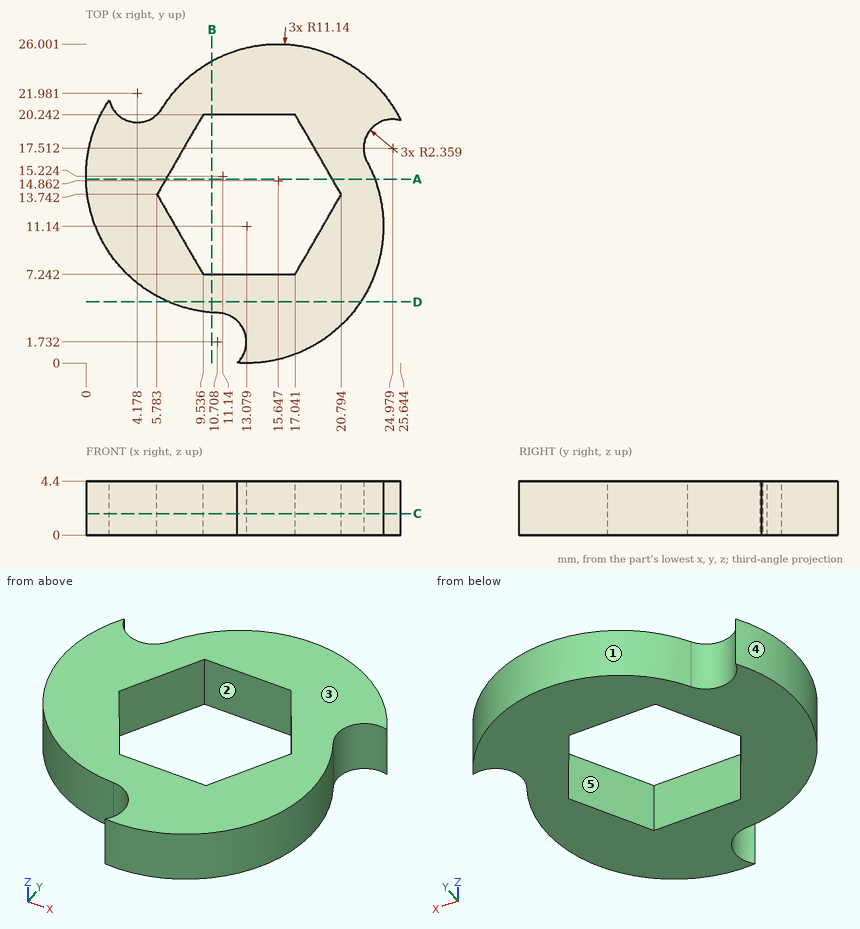
Drawing for the job (mm, zero at the part's lowest x, y, z). A direction names the side the tool comes from. Coordinates: 2 decimals unless noted, no trailing zeros. Order: outer loops, then holes, each group sorted by start corner. A loop starts at its lowest first (then second) coordinate and runs counter-clockwise, first axis right, second up. Notation, with made-up numbers: (51.5, 33.25) -> (55.5, 33.25) arc R11 ccw to (55.5, 50.25) -> close; hole circle Ø4 at (46, 22). An arc over 180 degrees is marked (long way). One line per item, written item: value.
(1) Slice it at B-B, the plane x = 10.25. List the corners of the cut face in (y, z).
Checked values:
outline: (4.12, 0) -> (7.24, 0) -> (7.24, 4.4) -> (4.12, 4.4) -> close; (20.24, 0) -> (24.61, 0) -> (24.61, 4.4) -> (20.24, 4.4) -> close
(2) Tool access for the marked faces 1 and 2: list every direction of +Z, -Z, +X, -X, +Y, -Y with a clear straight run to the whole face (end or side of a thin tool).
Checked values:
face 1: +Z, -Z, +Y
face 2: +Z, -Z
(3) Probe line 1 (Y direction, x = 16, z = 1) (1 decimal); line 2 (X direction, y = 12.5, z = 2.85) (1 decimal); line 3 (Y direction, x = 6, z = 0.9) (1 decimal). List the from-to ranges inside material, lowest first. Write a range as [from, to].
Checked values:
line 1: [0.4, 7.2], [20.2, 26]
line 2: [0.3, 6.5], [20.1, 24.1]
line 3: [5.3, 13.4], [14.1, 20.5]
(4) Slice it at D-D, the plane y = 5. List the corners of the cut face in (x, z) (1 decimal), plus the area to 3 significant figures.
Checked values:
outline: (6.7, 0) -> (22.4, 0) -> (22.4, 4.4) -> (6.7, 4.4) -> close
area: 68.9 mm2
(5) Slice it at C-C, the plane z = 1.75. List the corners of the cut face in (x, y) (1 decimal), plus the area to 3 significant figures.
Checked values:
outline: (1.9, 21.4) arc R11.1 ccw to (10.8, 4.1) arc R2.4 cw to (12.3, 0) arc R11.1 ccw to (22.9, 16.4) arc R2.4 cw to (25.6, 19.8) arc R11.1 ccw to (6.2, 20.7) arc R2.4 cw to start; hole (5.8, 13.7) -> (9.5, 7.2) -> (17, 7.2) -> (20.8, 13.7) -> (17, 20.2) -> (9.5, 20.2) -> close
area: 310 mm2
(6) Mould opens along Y. For the marked faces 3, 4 and 5 say: pulls with the +Y half, pulls with the -Y half, needs draft (parallel to the pull), parting line crosses it, or undercut.
Checked values:
face 3: needs draft
face 4: parting line crosses it
face 5: undercut
(7) Slice it at A-A, the plane y = 15. List the corners of the cut face in (x, z).
Checked values:
outline: (0, 0) -> (6.51, 0) -> (6.51, 4.4) -> (0, 4.4) -> close; (20.07, 0) -> (23.53, 0) -> (23.53, 4.4) -> (20.07, 4.4) -> close
(8) Drop flat-ended pins along their axis: pin 1 Ø2 at (y, z) = (7.5, 1) entering from -X; pin 2 Ø2 at (y, z) = (15.5, 2.5) entering from +X; pin 3 Ø8 at (x, y) = (8.5, 8.5) entering from -Z; pin 4 Ø1.3 at (x, z) = (11.5, 1.5) entering from -Y. Give the stop position or say it passes through.
Checked values:
pin 1: x = 2.26
pin 2: x = 23.7
pin 3: z = 0
pin 4: y = 3.6
